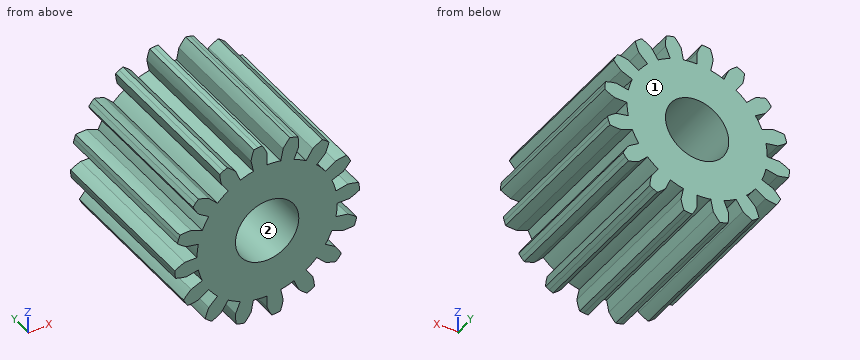
from build123d import *

# Parameters (mm, degrees)
F1_DEPTH = 6.35
F2_R     = 1.221512
F3_DEPTH = 30.89672


with BuildPart() as f1:
    # F0 (on Front) → F1 (new body)
    with BuildSketch(Plane.XZ):
        with BuildLine():
            Line((-1.763935, 2.639916), (-1.502873, 2.249208))
            ThreePointArc((-1.502873, 2.249208), (-1.716097, 2.091071), (-1.912795, 1.912795))
            Line((-1.912795, 1.912795), (-2.245064, 2.245064))
            ThreePointArc((-2.245064, 2.245064), (-2.445129, 2.326504), (-2.652293, 2.387669))
            Line((-2.652293, 2.387669), (-2.761528, 2.266327))
            Line((-2.761528, 2.266327), (-2.859227, 2.135519))
            ThreePointArc((-2.859227, 2.135519), (-2.758822, 1.944268), (-2.639916, 1.763935))
            Line((-2.639916, 1.763935), (-2.249208, 1.502873))
            ThreePointArc((-2.249208, 1.502873), (-2.385685, 1.275175), (-2.499187, 1.035197))
            Line((-2.499187, 1.035197), (-2.933318, 1.21502))
            ThreePointArc((-2.933318, 1.21502), (-3.149319, 1.213699), (-3.36412, 1.19093))
            Line((-3.36412, 1.19093), (-3.418605, 1.037022))
            Line((-3.418605, 1.037022), (-3.458809, 0.878784))
            ThreePointArc((-3.458809, 0.878784), (-3.292858, 0.740514), (-3.113993, 0.619412))
            Line((-3.113993, 0.619412), (-2.653122, 0.527739))
            ThreePointArc((-2.653122, 0.527739), (-2.692074, 0.265146), (-2.7051, 0))
            Line((-2.7051, 0), (-3.175, 0))
            ThreePointArc((-3.175, 0), (-3.374054, -0.08388), (-3.563791, -0.187118))
            Line((-3.563791, -0.187118), (-3.55523, -0.35016))
            Line((-3.55523, -0.35016), (-3.531819, -0.511739))
            ThreePointArc((-3.531819, -0.511739), (-3.325586, -0.575977), (-3.113993, -0.619412))
            Line((-3.113993, -0.619412), (-2.653122, -0.527739))
            ThreePointArc((-2.653122, -0.527739), (-2.588619, -0.785249), (-2.499187, -1.035197))
            Line((-2.499187, -1.035197), (-2.933318, -1.21502))
            ThreePointArc((-2.933318, -1.21502), (-3.08512, -1.36869), (-3.220907, -1.536678))
            Line((-3.220907, -1.536678), (-3.150604, -1.684033))
            Line((-3.150604, -1.684033), (-3.067141, -1.824353))
            ThreePointArc((-3.067141, -1.824353), (-2.852024, -1.80478), (-2.639916, -1.763935))
            Line((-2.639916, -1.763935), (-2.249208, -1.502873))
            ThreePointArc((-2.249208, -1.502873), (-2.091071, -1.716097), (-1.912795, -1.912795))
            Line((-1.912795, -1.912795), (-2.245064, -2.245064))
            ThreePointArc((-2.245064, -2.245064), (-2.326504, -2.445129), (-2.387669, -2.652293))
            Line((-2.387669, -2.652293), (-2.266327, -2.761528))
            Line((-2.266327, -2.761528), (-2.135519, -2.859227))
            ThreePointArc((-2.135519, -2.859227), (-1.944268, -2.758822), (-1.763935, -2.639916))
            Line((-1.763935, -2.639916), (-1.502873, -2.249208))
            ThreePointArc((-1.502873, -2.249208), (-1.275175, -2.385685), (-1.035197, -2.499187))
            Line((-1.035197, -2.499187), (-1.21502, -2.933318))
            ThreePointArc((-1.21502, -2.933318), (-1.213699, -3.149319), (-1.19093, -3.36412))
            Line((-1.19093, -3.36412), (-1.037022, -3.418605))
            Line((-1.037022, -3.418605), (-0.878784, -3.458809))
            ThreePointArc((-0.878784, -3.458809), (-0.740514, -3.292858), (-0.619412, -3.113993))
            Line((-0.619412, -3.113993), (-0.527739, -2.653122))
            ThreePointArc((-0.527739, -2.653122), (-0.265146, -2.692074), (0, -2.7051))
            Line((0, -2.7051), (0, -3.175))
            ThreePointArc((0, -3.175), (0.08388, -3.374054), (0.187118, -3.563791))
            Line((0.187118, -3.563791), (0.35016, -3.55523))
            Line((0.35016, -3.55523), (0.511739, -3.531819))
            ThreePointArc((0.511739, -3.531819), (0.575977, -3.325586), (0.619412, -3.113993))
            Line((0.619412, -3.113993), (0.527739, -2.653122))
            ThreePointArc((0.527739, -2.653122), (0.785249, -2.588619), (1.035197, -2.499187))
            Line((1.035197, -2.499187), (1.21502, -2.933318))
            ThreePointArc((1.21502, -2.933318), (1.36869, -3.08512), (1.536678, -3.220907))
            Line((1.536678, -3.220907), (1.684033, -3.150604))
            Line((1.684033, -3.150604), (1.824353, -3.067141))
            ThreePointArc((1.824353, -3.067141), (1.80478, -2.852024), (1.763935, -2.639916))
            Line((1.763935, -2.639916), (1.502873, -2.249208))
            ThreePointArc((1.502873, -2.249208), (1.716097, -2.091071), (1.912795, -1.912795))
            Line((1.912795, -1.912795), (2.245064, -2.245064))
            ThreePointArc((2.245064, -2.245064), (2.445129, -2.326504), (2.652293, -2.387669))
            Line((2.652293, -2.387669), (2.761528, -2.266327))
            Line((2.761528, -2.266327), (2.859227, -2.135519))
            ThreePointArc((2.859227, -2.135519), (2.758822, -1.944268), (2.639916, -1.763935))
            Line((2.639916, -1.763935), (2.249208, -1.502873))
            ThreePointArc((2.249208, -1.502873), (2.385685, -1.275175), (2.499187, -1.035197))
            Line((2.499187, -1.035197), (2.933318, -1.21502))
            ThreePointArc((2.933318, -1.21502), (3.149319, -1.213699), (3.36412, -1.19093))
            Line((3.36412, -1.19093), (3.418605, -1.037022))
            Line((3.418605, -1.037022), (3.458809, -0.878784))
            ThreePointArc((3.458809, -0.878784), (3.292858, -0.740514), (3.113993, -0.619412))
            Line((3.113993, -0.619412), (2.653122, -0.527739))
            ThreePointArc((2.653122, -0.527739), (2.692074, -0.265146), (2.7051, 0))
            Line((2.7051, 0), (3.175, 0))
            ThreePointArc((3.175, 0), (3.374054, 0.08388), (3.563791, 0.187118))
            Line((3.563791, 0.187118), (3.55523, 0.35016))
            Line((3.55523, 0.35016), (3.531819, 0.511739))
            ThreePointArc((3.531819, 0.511739), (3.325586, 0.575977), (3.113993, 0.619412))
            Line((3.113993, 0.619412), (2.653122, 0.527739))
            ThreePointArc((2.653122, 0.527739), (2.588619, 0.785249), (2.499187, 1.035197))
            Line((2.499187, 1.035197), (2.933318, 1.21502))
            ThreePointArc((2.933318, 1.21502), (3.08512, 1.36869), (3.220907, 1.536678))
            Line((3.220907, 1.536678), (3.150604, 1.684033))
            Line((3.150604, 1.684033), (3.067141, 1.824353))
            ThreePointArc((3.067141, 1.824353), (2.852024, 1.80478), (2.639916, 1.763935))
            Line((2.639916, 1.763935), (2.249208, 1.502873))
            ThreePointArc((2.249208, 1.502873), (2.091071, 1.716097), (1.912795, 1.912795))
            Line((1.912795, 1.912795), (2.245064, 2.245064))
            ThreePointArc((2.245064, 2.245064), (2.326504, 2.445129), (2.387669, 2.652293))
            Line((2.387669, 2.652293), (2.266327, 2.761528))
            Line((2.266327, 2.761528), (2.135519, 2.859227))
            ThreePointArc((2.135519, 2.859227), (1.944268, 2.758822), (1.763935, 2.639916))
            Line((1.763935, 2.639916), (1.502873, 2.249208))
            ThreePointArc((1.502873, 2.249208), (1.275175, 2.385685), (1.035197, 2.499187))
            Line((1.035197, 2.499187), (1.21502, 2.933318))
            ThreePointArc((1.21502, 2.933318), (1.213699, 3.149319), (1.19093, 3.36412))
            Line((1.19093, 3.36412), (1.037022, 3.418605))
            Line((1.037022, 3.418605), (0.878784, 3.458809))
            ThreePointArc((0.878784, 3.458809), (0.740514, 3.292858), (0.619412, 3.113993))
            Line((0.619412, 3.113993), (0.527739, 2.653122))
            ThreePointArc((0.527739, 2.653122), (0.265146, 2.692074), (0, 2.7051))
            Line((0, 2.7051), (0, 3.175))
            ThreePointArc((0, 3.175), (-0.08388, 3.374054), (-0.187118, 3.563791))
            Line((-0.187118, 3.563791), (-0.35016, 3.55523))
            Line((-0.35016, 3.55523), (-0.511739, 3.531819))
            ThreePointArc((-0.511739, 3.531819), (-0.575977, 3.325586), (-0.619412, 3.113993))
            Line((-0.619412, 3.113993), (-0.527739, 2.653122))
            ThreePointArc((-0.527739, 2.653122), (-0.785249, 2.588619), (-1.035197, 2.499187))
            Line((-1.035197, 2.499187), (-1.21502, 2.933318))
            ThreePointArc((-1.21502, 2.933318), (-1.36869, 3.08512), (-1.536678, 3.220907))
            Line((-1.536678, 3.220907), (-1.684033, 3.150604))
            Line((-1.684033, 3.150604), (-1.824353, 3.067141))
            ThreePointArc((-1.824353, 3.067141), (-1.80478, 2.852024), (-1.763935, 2.639916))
        make_face()
    extrude(amount=F1_DEPTH)

    # F2 (on Front) → F3 (cut)
    with BuildSketch(Plane.XZ):
        Circle(F2_R)
    extrude(amount=F3_DEPTH, mode=Mode.SUBTRACT)


solid = f1.part
The model under review builds one solid part; all positions refer to its coordinate system, in mm. Face numbers are marked on the shaded views. Round coordinates to 2 decimals unless told otherwise and drop trailing zeros. Answer as a JSON object with one key per item and string values.
Item 1: The part is to be moulded in two halves that separate along X. For the marked faces 1 and 2, say which applies: +X half, -X half, draft (parallel to the pull), parting line (faces both ways), or undercut.
Check sheet entries:
{"face 1": "draft", "face 2": "undercut"}
Item 2: Clearance check with flat-ended pins moving along their axes: P1, Ø3, axis at x = -2.5, y = -3.5, coming from the -Z side; P2, Ø2, axis at x = 0, z = 0, coming from the -Y side; P3, Ø1.5, axis at x = 3, y = -5.5, coming from the +Z side; P4, Ø0.5, axis at x = -3, y = -3, coming from the +Z side. State where each tip first meets the part, or that it passes through.
Check sheet entries:
{"P1": "z = -3.43", "P2": "through", "P3": "z = 2.77", "P4": "z = 2.28"}
Item 3: For line 1 along Z through (x, y) = (2.75, -1.5); line 2 along X through (y, z) = (-0.25, 2.75); line 3 along Z through (x, y) = (3, -1.25), list the stretches that pass through material, from the lowest coordinate up.
Check sheet entries:
{"line 1": "-2.28 to -1.93, -1.14 to -0.55, 0 to 0.55, 1.14 to 1.79", "line 2": "-1.79 to -1.14, -0.55 to 0, 0.55 to 1.14, 1.93 to 2.28", "line 3": "-1.22 to -0.6, 0 to 0.6, 1.28 to 1.82"}
